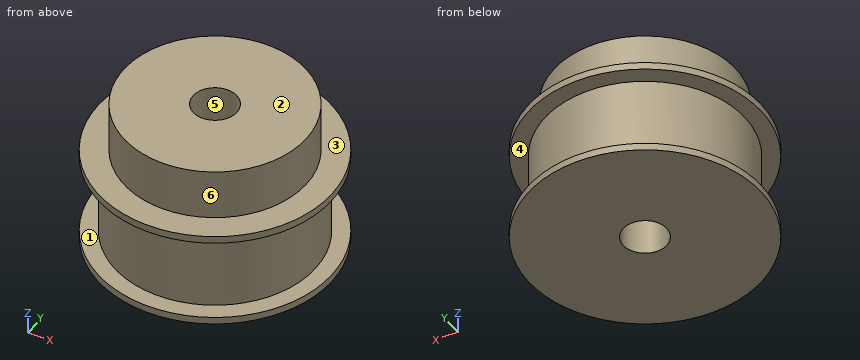
```python
from build123d import *

# Parameters (mm, degrees)
ESQUISSE1_R             = 13.75
BOSS_EXTRU_1_DEPTH      = 11.4
ESQUISSE2_R             = 16
BOSS_EXTRU_2_DEPTH      = 1
BOSS_EXTRU_3_START      = 1
ESQUISSE3_R             = 16
BOSS_EXTRU_3_DEPTH      = 1
ESQUISSE4_R             = 12.5
BOSS_EXTRU_4_DEPTH      = 7
ESQUISSE5_R             = 3
ENL_V_MAT_EXTRU_1_DEPTH = 30


with BuildPart() as part:
    # Esquisse1 → Boss.-Extru.1 (new body)
    with BuildSketch(Plane.XY):
        Circle(ESQUISSE1_R)
    extrude(amount=BOSS_EXTRU_1_DEPTH)

    # Esquisse2 → Boss.-Extru.2 (add)
    with BuildSketch(Plane.XY.offset(11.4)):
        Circle(ESQUISSE2_R)
    extrude(amount=BOSS_EXTRU_2_DEPTH)

    # Esquisse3 → Boss.-Extru.3 (add)
    with BuildSketch(Plane(origin=(0, 0, 0), x_dir=(-1, 0, 0), z_dir=(0, 0, -1)).offset(BOSS_EXTRU_3_START)):
        with Locations(Location((0, 0, 0), (0, 0, 180))):
            Circle(ESQUISSE3_R)
    extrude(amount=-BOSS_EXTRU_3_DEPTH)

    # Esquisse4 → Boss.-Extru.4 (add)
    with BuildSketch(Plane.XY.offset(12.4)):
        Circle(ESQUISSE4_R)
    extrude(amount=BOSS_EXTRU_4_DEPTH)

    # Esquisse5 → Enlèv. mat.-Extru.1 (cut)
    with BuildSketch(Plane(origin=(0, 0, -1), x_dir=(-1, 0, 0), z_dir=(0, 0, -1))):
        Circle(ESQUISSE5_R)
    extrude(amount=-ENL_V_MAT_EXTRU_1_DEPTH, mode=Mode.SUBTRACT)


solid = part.part
```
Work out the finished part from the listing and answer in its coordinate system (mm). Face numbers are marked on the shaded views. A direction names the side the tool comes from. Round coordinates to 2 decimals unless told otherwise and drop trailing zeros. Loops run counter-clockwise (first coordinate to the right, second up) from the corner with the lowest first, then second, coordinate; pieces in that order, holes last.
(1) Each of these flat-tipped pins is pushed along its axis until it touches: P1, Ø8, axis at y = -9, z = 16.5, coming from the +X side; P2, Ø5, axis at x = 0, y = 0, coming from the +Z side; P3, Ø2, axis at x = 11, z = 11.5, coming from the -Y side; P4, Ø6, axis at x = 2.5, z = 5.5, coming from the +Y side. Where does it stop, or does it pass through?
Computed values:
P1: stops at x = 11.46
P2: passes through
P3: stops at y = -12.49
P4: stops at y = 13.75
(2) Find the intervals of material crossed by L1, parallel to Z at x = -12, y = -9; L2, parallel to Y at x = 0, z = 3.5; L3, parallel to Z at x = -1.5, y = -13, in increasing order.
Computed values:
L1: z = -1 to 0, 11.4 to 12.4
L2: y = -13.75 to -3, 3 to 13.75
L3: z = -1 to 12.4
(3) The part is cut by section C-C, the plane x = 8. Give the vertices of the cut face in (y, z), and give its area (3 significant figures).
Computed values:
outline: (-13.86, -1) - (13.86, -1) - (13.86, 0) - (11.18, 0) - (11.18, 11.4) - (13.86, 11.4) - (13.86, 12.4) - (9.6, 12.4) - (9.6, 19.4) - (-9.6, 19.4) - (-9.6, 12.4) - (-13.86, 12.4) - (-13.86, 11.4) - (-11.18, 11.4) - (-11.18, 0) - (-13.86, 0) - close
area: 445 mm2
(4) For the marked faces 1, 2 and 3, determine the directions among +Z, -Z, +X, -X, +Y, -Y from which every point of the face is accessible in a straight line to the end or side of a thin tool.
Computed values:
face 1: none
face 2: +Z, +X, -X, +Y, -Y
face 3: +Z
(5) The mould has two halves that part along X. Classify the marked faces 4, 5 and 6: pulls with the +X half, pulls with the -X half, needs draft (parallel to the pull), parting line crosses it, or undercut.
Computed values:
face 4: needs draft
face 5: undercut
face 6: parting line crosses it
(6) The part is cut by section D-D, the plane y = -4. Give the vertices of the cut face in (x, z).
Computed values:
outline: (-15.49, -1) - (15.49, -1) - (15.49, 0) - (13.16, 0) - (13.16, 11.4) - (15.49, 11.4) - (15.49, 12.4) - (11.84, 12.4) - (11.84, 19.4) - (-11.84, 19.4) - (-11.84, 12.4) - (-15.49, 12.4) - (-15.49, 11.4) - (-13.16, 11.4) - (-13.16, 0) - (-15.49, 0) - close
(7) The part is cut by section A-A, the plane y = 0. Give the vertices of the cut face in (x, z).
Computed values:
outline: (-16, -1) - (-3, -1) - (-3, 19.4) - (-12.5, 19.4) - (-12.5, 12.4) - (-16, 12.4) - (-16, 11.4) - (-13.75, 11.4) - (-13.75, 0) - (-16, 0) - close; (3, -1) - (16, -1) - (16, 0) - (13.75, 0) - (13.75, 11.4) - (16, 11.4) - (16, 12.4) - (12.5, 12.4) - (12.5, 19.4) - (3, 19.4) - close
